```python
from build123d import *

# Parameters (mm, degrees)
F0_W     = 50
F0_H     = 50
F1_DEPTH = 300
F3_DEPTH = 50.001


with BuildPart() as f1:
    # F0 (on Top) → F1 (new body)
    with BuildSketch(Plane.XY):
        with Locations((25, 25)):
            Rectangle(F0_W, F0_H)
    extrude(amount=F1_DEPTH)

    # F2 (on face) → F3 (cut, through all)
    with BuildSketch(Plane(origin=(0, 50, 0), x_dir=(-1, 0, 0), z_dir=(0, 1, 0))):
        with BuildLine():
            Line((-50, 210), (-45, 210))
            ThreePointArc((-45, 210), (-39, 216), (-45, 222))
            Line((-45, 222), (-50, 222))
            Line((-50, 222), (-50, 210))
        make_face()
        with BuildLine():
            Line((0, 222), (-5, 222))
            ThreePointArc((-5, 222), (-11, 216), (-5, 210))
            Line((-5, 210), (0, 210))
            Line((0, 210), (0, 222))
        make_face()
        with BuildLine():
            Line((-50, 110), (-45, 110))
            ThreePointArc((-45, 110), (-39, 116), (-45, 122))
            Line((-45, 122), (-50, 122))
            Line((-50, 122), (-50, 110))
        make_face()
        with BuildLine():
            Line((0, 122), (-5, 122))
            ThreePointArc((-5, 122), (-11, 116), (-5, 110))
            Line((-5, 110), (0, 110))
            Line((0, 110), (0, 122))
        make_face()
    extrude(amount=-F3_DEPTH, mode=Mode.SUBTRACT)


solid = f1.part
```
Input: part model. Units: mm. Frame: model coordinates. A direction names the side the tool comes from. Coordinates: 2 decimals unless noted, no trailing zeros. Loops run counter-clockwise (first coordinate to the right, second up) from the corner with the lowest first, then second, coordinate; pieces in that order, holes last.
Q1. Section A-A, the plane y = 7.5. Return the cut outline in (x, z), and give its area (3 significant figures).
Results are:
outline: (0, 0) - (50, 0) - (50, 110) - (45, 110) arc R6 cw to (45, 122) - (50, 122) - (50, 210) - (45, 210) arc R6 cw to (45, 222) - (50, 222) - (50, 300) - (0, 300) - (0, 222) - (5, 222) arc R6 cw to (5, 210) - (0, 210) - (0, 122) - (5, 122) arc R6 cw to (5, 110) - (0, 110) - close
area: 14,500 mm2
Q2. Line query: line 1 along Z through (x, y) = (4, 4.5); line 2 along Z through (x, y) = (41.5, 7.5). Output: solid intervals per line, ascending.
Results are:
line 1: z = 0 to 110, 122 to 210, 222 to 300
line 2: z = 0 to 111.13, 120.87 to 211.13, 220.87 to 300
Q3. Section B-B, the plane z = 216. Return the cut outline in (x, y), and give its area (3 significant figures).
Results are:
outline: (11, 0) - (39, 0) - (39, 50) - (11, 50) - close
area: 1,400 mm2
Q4. Contact query for a flat-ended pin moving along its axis: pin 1 (1 mm diameter, centred on y = 36, z = 216.5, fed in from +X). Output: stop coordinate, or through.
Results are:
pin 1: stops at x = 39.08
Q5. Mould query, pull axis Z, two halves, no side actions, for faces 1 (the flat face through (50, 25, 260)), 2 (the flat face through (25, 25, 300)), 3 (the flat face through (3, 25, 110)). Classes: +Z half, -Z half, draft (parallel to the pull), parting line (faces both ways), or undercut.
Results are:
face 1: draft
face 2: +Z half
face 3: undercut
Q6. Set-up query: faces 4 (the flat face through (48, 25, 210)), 5 (the flat face through (25, 25, 0)), 6 (the flat face through (2, 25, 222)). Return all of +Z, -Z, +X, -X, +Y, -Y with unobstructed straight access to the full face (end or side cutting, diameter ignored); none if empty.
Results are:
face 4: +X, +Y, -Y
face 5: -Z, +X, -X, +Y, -Y
face 6: -X, +Y, -Y
